Geometry check sheet. Reference: the model listing, model coordinates, mm. A direction names the side the tool comes from. Give positions to 0.01 mm unless a question says otherwise; leave off trailing zeros. Write each loop counter-clockwise with the first axis right and the second up, starting at its lowest first coordinate (ties: lowest second). Pieces come first, ordered by that corner, then holes. Notation, with made-up numbers: (-23.5, 20) -> (29.5, 20) arc R32 cw to (29.5, 53) -> close; hole circle Ø8 at (71, 64.25). An arc over 180 degrees is marked (long way). Use a Markdown table: item, result. Add a question column.
from build123d import *

# Parameters (mm, degrees)
SKETCH1_W           = 40.3
SKETCH1_H           = 20.1
BOSS_EXTRUDE1_DEPTH = 40.25
SKETCH2_R           = 2.9
BOSS_EXTRUDE2_DEPTH = 6.2
BOSS_EXTRUDE3_START = -5
SKETCH3_W           = 6.65
SKETCH3_H           = 20.1
SKETCH3_R           = 2
BOSS_EXTRUDE3_DEPTH = 2.5


with BuildPart() as part:
    # Sketch1 → Boss-Extrude1 (new body)
    with BuildSketch(Plane(origin=(0, 0, 0), x_dir=(1, 0, 0), z_dir=(0, 1, 0))):
        Rectangle(SKETCH1_W, SKETCH1_H)
    extrude(amount=BOSS_EXTRUDE1_DEPTH)

    # Sketch2 → Boss-Extrude2 (add)
    with BuildSketch(Plane(origin=(0, 40.25, 0), x_dir=(1, 0, 0), z_dir=(0, 1, 0))):
        with Locations(Location((10.15, 0, 0), (0, 0, 90))):
            Circle(SKETCH2_R)
    extrude(amount=BOSS_EXTRUDE2_DEPTH)

    # Sketch3 → Boss-Extrude3 (add)
    # profile 1 of 2: a face of its own
    with BuildSketch(Plane(origin=(0, 40.25, 0), x_dir=(1, 0, 0), z_dir=(0, 1, 0)).offset(BOSS_EXTRUDE3_START)):
        with Locations((-23.475, 0)):
            Rectangle(SKETCH3_W, SKETCH3_H)
        with Locations(Location((-24.794421729, 5.55, 0), (0, 0, 270))):
            Circle(SKETCH3_R, mode=Mode.SUBTRACT)
        with Locations(Location((-24.794421729, -5.55, 0), (0, 0, 270))):
            Circle(SKETCH3_R, mode=Mode.SUBTRACT)
    # profile 2 of 2: a face of its own
    with BuildSketch(Plane(origin=(0, 40.25, 0), x_dir=(1, 0, 0), z_dir=(0, 1, 0)).offset(BOSS_EXTRUDE3_START)):
        with Locations((23.475, 0)):
            Rectangle(SKETCH3_W, SKETCH3_H)
        with Locations(Location((24.794421729, -5.55, 0), (0, 0, 270))):
            Circle(SKETCH3_R, mode=Mode.SUBTRACT)
        with Locations(Location((24.794421729, 5.55, 0), (0, 0, 270))):
            Circle(SKETCH3_R, mode=Mode.SUBTRACT)
    extrude(amount=-BOSS_EXTRUDE3_DEPTH)


solid = part.part
1) Gauge pin test, flat ends, axial feed: P1, Ø6, axis at x = -2.5, z = 1.5, coming from the +Y side; P2, Ø10, axis at y = 15, z = -2.5, coming from the +X side; P3, Ø1.5, axis at y = 39.5, z = -7.5, coming from the -X side; P4, Ø3, axis at x = 24.79, z = -5.55, coming from the -Y side. Record the tip position at first contact, or that the pin passes through.
2) Tool access check on faces 1 (the face through (7.275, 43.307, 0.378)), 2 (the face through (-23, 32.75, 0)), 3 (the face through (23, 32.75, 0)), 4 (the face through (20.15, 38, 0)), 5 (the face through (-20.15, 38, 0)). Record the directions out of +Z, -Z, +X, -X, +Y, -Y that give a thin tool (end or side, any length) a straight path to the whole face; none if there is none.
3) Material ranges on probe 1 along Y at (x, z) = (0.5, -8.5); probe 2 along X at (y, z) = (8.5, -3.75); probe 3 along Y at (x, z) = (-23, -3.25), recorded low to high. Write a range as [from, to].
4) Sectioned sample at C-C, the plane x = 10.15. Enter the section's corners in (y, z), and give its area (3 significant figures).
5) Draft check along X on faces 6 (the face through (-26.8, 34, 0)), 7 (the face through (-26.57, 34.02, -4.63)), 8 (the face through (0, 20, -10.05)), 9 (the face through (26.48, 34.02, 6.63)). Enter one of: +X half, -X half, draft (parallel to the pull), parting line (faces both ways), or undercut.
6) Sectioned sample at B-B, the plane z = 8.75. Enter the section's corners in (x, y).
7) Sectioned sample at D-D, the plane y = 33.5. Enter the section's corners in (x, z).
8) Sectioned sample at A-A, the plane z = 5.55. Count the separate pieces of the cut face and the enclosed holes in it, and give its area (3 significant figures).
Check values:
| question | item | result |
|---|---|---|
| 1 | P1 | y = 40.25 |
| 1 | P2 | x = 20.15 |
| 1 | P3 | x = -20.15 |
| 1 | P4 | through |
| 2 | face 1 | +Y |
| 2 | face 2 | +Z, -Z, -X, -Y |
| 2 | face 3 | +Z, -Z, +X, -Y |
| 2 | face 4 | +Z, -Z, +X, +Y |
| 2 | face 5 | +Z, -Z, -X, +Y |
| 3 | probe 1 | [0, 40.25] |
| 3 | probe 2 | [-20.15, 20.15] |
| 3 | probe 3 | [32.75, 35.25] |
| 4 | outline | (0, -10.05) -> (40.25, -10.05) -> (40.25, -2.9) -> (46.45, -2.9) -> (46.45, 2.9) -> (40.25, 2.9) -> (40.25, 10.05) -> (0, 10.05) -> close |
| 4 | area | 845 mm² |
| 5 | face 6 | -X half |
| 5 | face 7 | undercut |
| 5 | face 8 | draft |
| 5 | face 9 | undercut |
| 6 | outline | (-26.8, 32.75) -> (-20.15, 32.75) -> (-20.15, 0) -> (20.15, 0) -> (20.15, 32.75) -> (26.8, 32.75) -> (26.8, 35.25) -> (20.15, 35.25) -> (20.15, 40.25) -> (-20.15, 40.25) -> (-20.15, 35.25) -> (-26.8, 35.25) -> close |
| 7 | outline | (-26.8, -10.05) -> (26.8, -10.05) -> (26.8, 10.05) -> (-26.8, 10.05) -> close; hole circle Ø4 at (-24.79, -5.55); hole circle Ø4 at (-24.79, 5.55); hole circle Ø4 at (24.79, -5.55); hole circle Ø4 at (24.79, 5.55) |
| 8 | separate pieces | 3 |
| 8 | enclosed holes | 0 |
| 8 | area | 1,640 mm² |
